Could you check a few things on this model? Use its own coordinates, in mm. Face numbers are marked on the shaded views. Give positions to 0.01 mm unless a question says otherwise; leave off trailing zeros. Order: outer loops, then holes, each group sorted by start corner. A loop starts at its lowest first (then second) coordinate and runs counter-clockwise, first axis right, second up. Notation, with made-up numbers: (86, 2) -> (139, 2) arc R14 cw to (139, 8) -> close; hole circle Ø11 at (38, 62.5). An arc over 180 degrees is marked (long way). One line per item, written item: value.
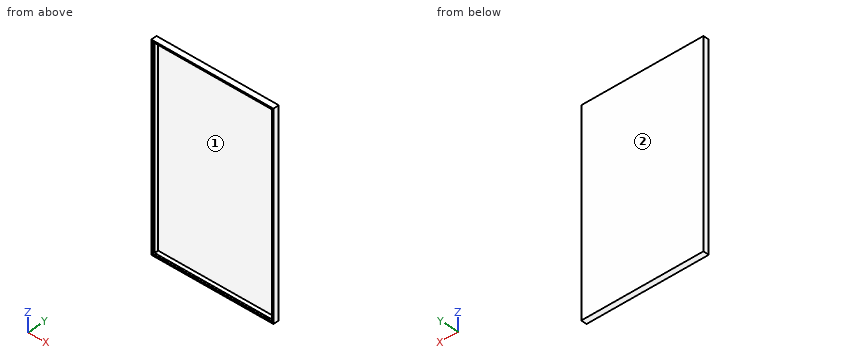
```python
from build123d import *

# Parameters (mm, degrees)
F0_W     = 3
F0_H     = 1044
F1_DEPTH = 30
F2_W     = 634
F2_H     = 1044
F3_DEPTH = 5
F4_W     = 10
F4_H     = 1024
F5_DEPTH = 20


with BuildPart() as f1:
    # F0 (on Front) → F1 (new body)
    with BuildSketch(Plane.XZ):
        Polygon((-634, 0), (0, 0), (3, 0), (3, 3), (-637, 3), (-637, 0), align=None)
        with Locations((1.5, -522)):
            Rectangle(F0_W, F0_H)
        with Locations((-635.5, -522)):
            Rectangle(F0_W, F0_H)
        Polygon((3, -1044), (0, -1044), (-634, -1044), (-637, -1044), (-637, -1047), (3, -1047), align=None)
    extrude(amount=F1_DEPTH)

    # F2 (on Front) → F3 (join)
    with BuildSketch(Plane.XZ):
        with Locations((-317, -522)):
            Rectangle(F2_W, F2_H)
    extrude(amount=F3_DEPTH)

    # F4 (on face) → F5 (join)
    with BuildSketch(Plane.XZ.offset(5)):
        Polygon((0, -10), (0, 0), (-634, 0), (-634, -10), (-624, -10), (-10, -10), align=None)
        with Locations((-629, -522)):
            Rectangle(F4_W, F4_H)
        Polygon((0, -1044), (0, -1034), (-10, -1034), (-624, -1034), (-634, -1034), (-634, -1044), align=None)
        with Locations((-5, -522)):
            Rectangle(F4_W, F4_H)
    extrude(amount=F5_DEPTH)


solid = f1.part
```
1) We'd pull the mould along Z, two halves only. Please class the marked faces 1 and 2: +Z half, -Z half, draft (parallel to the pull), parting line (faces both ways), or undercut.
Answer below:
face 1: undercut
face 2: draft
2) Suppose I cut it at B-B, the plane z = -337. Write out the boundary of the cut face in (x, y), then the cut area to 3 significant figures.
Answer below:
outline: (-637, -30) -> (-634, -30) -> (-634, -25) -> (-624, -25) -> (-624, -5) -> (-10, -5) -> (-10, -25) -> (0, -25) -> (0, -30) -> (3, -30) -> (3, 0) -> (-637, 0) -> close
area: 3,750 mm2
3) If I drill on line 1 along X through (y, z) = (-14.75, -745.5); line 2 along Z through (x, y) = (-225.5, -14.5); line 3 along X through (y, z) = (-28.25, -751), over which ranges is the centre line in solid material (lowest first)?
Answer below:
line 1: x = -637 to -624, -10 to 3
line 2: z = -1047 to -1034, -10 to 3
line 3: x = -637 to -634, 0 to 3
4) Suppose I cut it at A-A, the plane y = -15.75. Write out the boundary of the cut face in (x, z), then the cut area to 3 significant figures.
Answer below:
outline: (-637, -1047) -> (3, -1047) -> (3, 3) -> (-637, 3) -> close; hole (-624, -1034) -> (-10, -1034) -> (-10, -10) -> (-624, -10) -> close
area: 43,300 mm2
5) Suppose I cut it at C-C, the plane x = -133.5. Write out the boundary of the cut face in (y, z), then the cut area to 3 significant figures.
Answer below:
outline: (-30, -1047) -> (0, -1047) -> (0, 3) -> (-30, 3) -> (-30, 0) -> (-25, 0) -> (-25, -10) -> (-5, -10) -> (-5, -1034) -> (-25, -1034) -> (-25, -1044) -> (-30, -1044) -> close
area: 5,800 mm2
